The listing builds one solid part. Answer for the finished solid, in the listing's coordinates (mm). Face numbers are marked on the shaded views. Coordinates: 2 decimals unless noted, no trailing zeros. Order: outer loops, then holes, each group sorted by start corner. A loop starts at its lowest first (then second) coordinate and runs counter-clockwise, first axis right, second up. Notation, with made-up numbers: (67.5, 70) -> (84.5, 70) arc R10 ccw to (84.5, 86) -> close; hole circle Ø11 at (83, -12). An arc over 180 degrees is marked (long way). Write item = value, one per line.
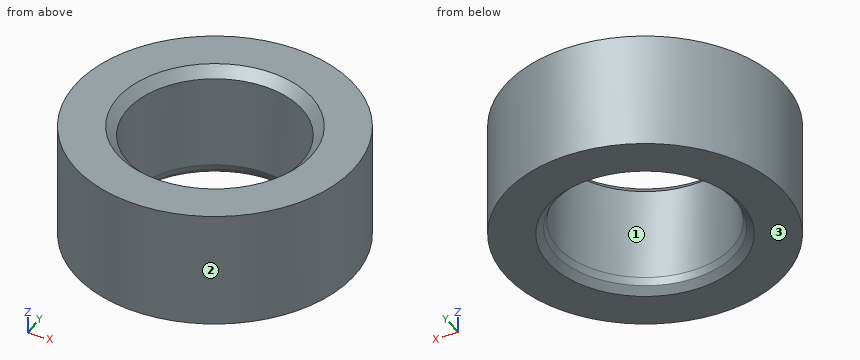
from build123d import *

# Parameters (mm, degrees)
F0_R     = 7.2
F0_R_2   = 4.5
F1_DEPTH = 6
F2_SIZE2 = 0.5
F2_SIZE  = 0.5


# Not quite as in the source:
# - a fillet or chamfer that OpenCascade refuses, or shapes differently, is made with other operations: its cross-section is extruded or revolved along the edge and cut away or added


with BuildPart() as f1:
    # F0 (on Top) → F1 (new body)
    with BuildSketch(Plane.XY):
        Circle(F0_R)
        Circle(F0_R_2, mode=Mode.SUBTRACT)
    extrude(amount=F1_DEPTH)

    # F2
    f2_edges = [f1.edges().sort_by_distance(p)[0] for p in [
        (-4.5, 0, 0),
    ]]
    chamfer(f2_edges, length=F2_SIZE, length2=F2_SIZE2)

    # F3: chamfer of 0.5 on 3 edges, made by hand

    # F3_s1 → F3_t2 (revolve, cut)
    with BuildSketch(Plane.XZ):
        Polygon((4.5, 0.7071067812), (4.6464466094, 0.3535533906), (4.5, 0.5), align=None)
    revolve(axis=Axis((0, 0, 0.5), (0, 0, 1)), mode=Mode.SUBTRACT)

    # F3_s3 → F3_t4 (revolve, cut)
    with BuildSketch(Plane.XZ):
        Polygon((4.5, 5.5), (5, 6), (4.5, 6), align=None)
    revolve(axis=Axis((0, 0, 6), (0, 0, 1)), mode=Mode.SUBTRACT)


solid = f1.part
Q1. Section D-D, the plane x = -6 is taken. Give the vertices of the cut face in (y, z), plus the area to 3 significant figures.
The answers:
outline = (-3.98, 0) -> (3.98, 0) -> (3.98, 6) -> (-3.98, 6) -> close
area = 47.8 mm2
Q2. Section C-C, the plane z = 3.35 is taken. Give the vertices of the cut face in (x, y), plus the area to 3 significant figures.
The answers:
outline = circle Ø14.4 at (0, 0); hole circle Ø9 at (0, 0)
area = 99.2 mm2
Q3. The mould has two halves that part along Y. Classify the marked faces 1, 2 and 3: released by +Y, released by -Y, zero draft, split by the parting line, or undercut.
The answers:
face_1 = undercut
face_2 = split by the parting line
face_3 = zero draft
Q4. Each of these flat-tipped pins is pushed along its axis until it touches: pin 1 Ø3 at (y, z) = (-0.5, 5) entering from -X; pin 2 Ø1 at (y, z) = (-5, 5) entering from +X; pin 3 Ø1.5 at (x, z) = (-1.5, 1.5) entering from -Y; pin 4 Ø6 at (x, y) = (0, 0) entering from -Z. Where does it stop, or does it pass through?
The answers:
pin_1 = -7.2
pin_2 = 5.62
pin_3 = -7.16
pin_4 = through
Q5. Section A-A, the plane x = 0 is taken. Give the vertices of the cut face in (y, z), plus the area to 3 significant figures.
The answers:
outline = (-7.2, 0) -> (-5, 0) -> (-4.65, 0.35) -> (-4.5, 0.71) -> (-4.5, 5.5) -> (-5, 6) -> (-7.2, 6) -> close; (4.5, 0.71) -> (4.65, 0.35) -> (5, 0) -> (7.2, 0) -> (7.2, 6) -> (5, 6) -> (4.5, 5.5) -> close
area = 31.9 mm2
Q6. Find the intervals of material crossed by line 1 along Y through (x, z) = (0, 3.1); line 2 along Y through (x, z) = (2.5, 3.3); line 3 along X through (y, z) = (-3, 4.95), in increasing order.
The answers:
line_1 = -7.2 to -4.5, 4.5 to 7.2
line_2 = -6.75 to -3.74, 3.74 to 6.75
line_3 = -6.55 to -3.35, 3.35 to 6.55
